from build123d import *

# Parameters (mm, degrees)
SKETCH1_W               = 76.2
SKETCH1_H               = 44.45
BOSS_EXTRUDE1_DEPTH     = 9.525
F_10_32_TAPPED_HOLE1_D  = 4.0386
SKETCH9_R               = 7.366
BOSS_EXTRUDE2_DEPTH     = 1.397
F_3_8_16_TAPPED_HOLE1_D = 7.9375


with BuildPart() as part:
    # Sketch1 → Boss-Extrude1 (new body)
    with BuildSketch(Plane(origin=(0, 0, 0), x_dir=(1, 0, 0), z_dir=(0, 1, 0))):
        with Locations((38.1, 22.225)):
            Rectangle(SKETCH1_W, SKETCH1_H)
    extrude(amount=BOSS_EXTRUDE1_DEPTH)

    # #10-32 Tapped Hole1 (through all)
    with Locations(Plane(origin=(0, 9.525, 0), x_dir=(-1, 0, 0), z_dir=(0, 1, 0))):
        with Locations((-6.35, -38.1), (-69.85, -38.1), (-69.85, -6.35), (-6.35, -6.35)):
            Hole(F_10_32_TAPPED_HOLE1_D / 2)

    # Sketch9 → Boss-Extrude2 (add)
    with BuildSketch(Plane(origin=(0, 9.525, 0), x_dir=(1, 0, 0), z_dir=(0, 1, 0))):
        with Locations(Location((38.1, 22.225, 0), (0, 0, 90))):
            Circle(SKETCH9_R)
    extrude(amount=BOSS_EXTRUDE2_DEPTH)

    # 3/8-16 Tapped Hole1 (through all)
    with Locations(Plane(origin=(0, 10.922, 0), x_dir=(-1, 0, 0), z_dir=(0, 1, 0))):
        with Locations((-38.1, -22.225)):
            Hole(F_3_8_16_TAPPED_HOLE1_D / 2)


solid = part.part
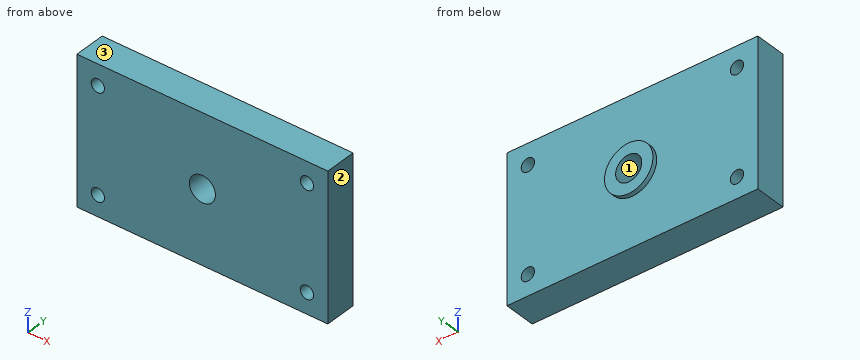
Here's how the part is built. I have some questions about the finished solid (model axes, mm). Face numbers are marked on the shaded views. Coordinates: 2 decimals unless noted, no trailing zeros. Order: outer loops, then holes, each group sorted by start corner. A loop starts at its lowest first (then second) coordinate and runs counter-clockwise, first axis right, second up. Notation, with made-up numbers: (52.5, -27.75) - (79.5, -27.75) arc R10 cw to (79.5, -22.75) - close; hole circle Ø10 at (83.25, 81.25). An arc over 180 degrees is marked (long way). Use CSV: the item, a comma, the result in double quotes. Start each with the question number.
1. Suppose I cut it at D-D on y = 1. Give the number of separate pieces and of enclosed holes in the cut face, then the cut area to 3 significant figures.
2. Suppose I cut it at C-C on x = 38.1. List the corners of the cut face in (y, z) for me (3 decimals), then the cut area to 3 significant figures.
3. Suppose I cut it at A-A on z = -38.1. List the corners of the cut face in (x, y) for me (3 decimals).
4. If we mould it in two halves opening along X, with no side actions, what happens to the marked faces 1, 2 and 3? For each: +X half, -X half, draft (parallel to the pull), parting line (faces both ways), or undercut.
5. I'm going to push flat-ended pins straight in: pin 1 (3.5 mm diameter, centred on x = 6.35, z = -38.1, fed in from -Y); pin 2 (1 mm diameter, centred on x = 27, y = 7, fed in from +Z); pin 3 (2 mm diameter, centred on x = 41, z = -37.5, fed in from +Y) (3 decimals). Where does each tip first touch, or does it pass through?
6. Please list where these lines run through material, in increasing order: line 1 (Z direction, x = 69.85, y = 2.5); line 2 (X direction, y = 7, z = -6.5); line 3 (X direction, y = 6.25, z = -39.5). Write a range as from..to.
7. Suppose I cut it at B-B on x = 6.35. List the corners of the cut face in (y, z) for me (3 decimals), then the cut area to 3 significant figures.
Output:
1,separate pieces,"1"
1,enclosed holes,"5"
1,area,"3,290 mm2"
2,outline,"(0, -44.45) - (9.525, -44.45) - (9.525, -29.591) - (10.922, -29.591) - (10.922, -26.194) - (0, -26.194) - close; (0, -18.256) - (10.922, -18.256) - (10.922, -14.859) - (9.525, -14.859) - (9.525, 0) - (0, 0) - close"
2,area,"357 mm2"
3,outline,"(0, 0) - (4.331, 0) - (4.331, 9.525) - (0, 9.525) - close; (8.369, 0) - (67.831, 0) - (67.831, 9.525) - (8.369, 9.525) - close; (71.869, 0) - (76.2, 0) - (76.2, 9.525) - (71.869, 9.525) - close"
4,face 1,"undercut"
4,face 2,"+X half"
4,face 3,"draft"
5,pin 1,"passes through"
5,pin 2,"stops at z = 0"
5,pin 3,"stops at y = 9.525"
6,line 1,"z = -44.45..-40.12, -36.08..-8.37, -4.33..0"
6,line 2,"x = 0..4.34, 8.36..67.84, 71.86..76.2"
6,line 3,"x = 0..4.89, 7.81..68.39, 71.31..76.2"
7,outline,"(0, -44.45) - (9.525, -44.45) - (9.525, -40.119) - (0, -40.119) - close; (0, -36.081) - (9.525, -36.081) - (9.525, -8.369) - (0, -8.369) - close; (0, -4.331) - (9.525, -4.331) - (9.525, 0) - (0, 0) - close"
7,area,"346 mm2"
